from build123d import *

# Parameters (mm, degrees)
ESQUISSE1_W             = 45
ESQUISSE1_H             = 250
BOSS_EXTRU_2_DEPTH      = 3
ESQUISSE2_W             = 3
ESQUISSE2_H             = 250
BOSS_EXTRU_3_DEPTH      = 90
ESQUISSE3_W             = 83
ESQUISSE3_H             = 250
BOSS_EXTRU_4_DEPTH      = 3
ESQUISSE4_R             = 10
ESQUISSE4_R_2           = 2.5
ESQUISSE4_R_3           = 2
ENL_V_MAT_EXTRU_1_DEPTH = 3
ESQUISSE5_R             = 1.5
ENL_V_MAT_EXTRU_2_DEPTH = 3
ENL_V_START             = -3
ESQUISSE6_R             = 10
ESQUISSE6_R_2           = 2
ESQUISSE6_R_3           = 2.5
ENL_V_MAT_EXTRU_3_DEPTH = 3


with BuildPart() as part:
    # Esquisse1 → Boss.-Extru.2 (new body)
    with BuildSketch(Plane.XY):
        with Locations((-2.435511103, -80.979780034)):
            Rectangle(ESQUISSE1_W, ESQUISSE1_H)
    boss_extru_2 = extrude(amount=BOSS_EXTRU_2_DEPTH)

    # Esquisse2 → Boss.-Extru.3 (add)
    with BuildSketch(Plane.XY.offset(3)):
        with Locations((-23.435511103, -80.979780034)):
            Rectangle(ESQUISSE2_W, ESQUISSE2_H)
    boss_extru_3 = extrude(amount=BOSS_EXTRU_3_DEPTH)

    # Esquisse3 → Boss.-Extru.4 (add)
    with BuildSketch(Plane.XY.offset(93)):
        with Locations((-63.435511103, -80.979780034)):
            Rectangle(ESQUISSE3_W, ESQUISSE3_H)
    boss_extru_4 = extrude(amount=BOSS_EXTRU_4_DEPTH)

    # Esquisse4 → Enl_v. mat.-Extru.1 (cut)
    with BuildSketch(Plane.ZY.offset(24.935511103)):
        with Locations(Location((30.5, -80.979780034, 0), (0, 0, 270))):
            Circle(ESQUISSE4_R)
        with Locations(Location((30.5, -59.979780034, 0), (0, 0, 270))):
            Circle(ESQUISSE4_R_2)
        with Locations(Location((48.686533479, -91.479780034, 0), (0, 0, 270))):
            Circle(ESQUISSE4_R_2)
        with Locations(Location((30.5, -0.979780034, 0), (0, 0, 270))):
            Circle(ESQUISSE4_R_3)
        with Locations(Location((30.5, -160.979780034, 0), (0, 0, 270))):
            Circle(ESQUISSE4_R_2)
        with Locations(Location((12.313466521, -91.479780034, 0), (0, 0, 270))):
            Circle(ESQUISSE4_R_2)
    extrude(amount=-ENL_V_MAT_EXTRU_1_DEPTH, mode=Mode.SUBTRACT)

    # Esquisse5 → Enl_v. mat.-Extru.2 (cut)
    with BuildSketch(Plane.XY.offset(96)):
        with BuildLine():
            ThreePointArc((-99.435511103, -80.979780034), (-100.935511103, -79.479780034), (-102.435511103, -80.979780034))
            Line((-102.435511103, -80.979780034), (-99.435511103, -80.979780034))
        make_face()
        with BuildLine():
            Line((-99.435511103, -80.979780034), (-102.435511103, -80.979780034))
            ThreePointArc((-102.435511103, -80.979780034), (-100.935511103, -82.479780034), (-99.435511103, -80.979780034))
        make_face()
        with Locations((-100.935511103, -165.979780034)):
            Circle(ESQUISSE5_R)
        with Locations((-100.935511103, 4.020219966)):
            Circle(ESQUISSE5_R)
    enl_v_mat_extru_2 = extrude(amount=-ENL_V_MAT_EXTRU_2_DEPTH, mode=Mode.SUBTRACT)

    # Sym_trie1: Boss.-Extru.2, Boss.-Extru.3, Boss.-Extru.4, Enl_v. mat.-Extru.2 across plane
    add(boss_extru_2.mirror(Plane(origin=(20.064488897, 44.020219966, 3), x_dir=(0, 0, 1), z_dir=(1, 0, 0))))
    add(boss_extru_3.mirror(Plane(origin=(20.064488897, 44.020219966, 3), x_dir=(0, 0, 1), z_dir=(1, 0, 0))))
    add(boss_extru_4.mirror(Plane(origin=(20.064488897, 44.020219966, 3), x_dir=(0, 0, 1), z_dir=(1, 0, 0))))
    add(enl_v_mat_extru_2.mirror(Plane(origin=(20.064488897, 44.020219966, 3), x_dir=(0, 0, 1), z_dir=(1, 0, 0))), mode=Mode.SUBTRACT)

    # Esquisse6 → Enl_v. mat.-Extru.3 (cut)
    with BuildSketch(Plane(origin=(65.064488897, 0, 0), x_dir=(0, 0, -1), z_dir=(1, 0, 0)).offset(ENL_V_START)):
        with Locations(Location((-30.5, -80.979780034, 0), (0, 0, 270))):
            Circle(ESQUISSE6_R)
        with Locations(Location((-30.5, -0.979780034, 0), (0, 0, 270))):
            Circle(ESQUISSE6_R_2)
        with Locations(Location((-30.5, -160.979780034, 0), (0, 0, 270))):
            Circle(ESQUISSE6_R_3)
        with Locations(Location((-30.5, -101.979780034, 0), (0, 0, 90))):
            Circle(ESQUISSE6_R_3)
        with Locations(Location((-48.686533479, -70.479780034, 0), (0, 0, 90))):
            Circle(ESQUISSE6_R_3)
        with Locations(Location((-12.313466521, -70.479780034, 0), (0, 0, 90))):
            Circle(ESQUISSE6_R_3)
    extrude(amount=ENL_V_MAT_EXTRU_3_DEPTH, mode=Mode.SUBTRACT)


solid = part.part
Can you work these out from the model? Positions are in its coordinate system, mm. A direction names the side the tool comes from. Round coordinates to 2 decimals unless told otherwise and drop trailing zeros. Write each loop counter-clockwise with the first axis right and the second up, starting at its lowest first coordinate (ties: lowest second). Pieces come first, ordered by that corner, then holes. Notation, with made-up numbers: (16, 36.5) -> (43, 36.5) arc R11 ccw to (43, 55.5) -> close; hole circle Ø5 at (71.25, 9). An arc over 180 degrees is marked (long way). Use one line per item in the form item = value. Start each with the question number.
Q1. Imagine slicing it at C-C (x = -81.5). Please give me the cut outline in (y, z), then the cut area to 3 significant figures.
Q2. Imagine slicing it at A-A (z = 84). Please give me the cut outline in (x, y).
Q3. I'm going to push flat-ended pins straight in: P1, Ø6, axis at y = -91.48, z = 12.31, coming from the -X side; P2, Ø10, axis at x = -76, y = -59.5, coming from the -Z side; P3, Ø4.5, axis at y = -59.98, z = 30.5, coming from the -X side; P4, Ø2.5, axis at x = -100.94, y = -165.98, coming from the -Z side. Where does each tip first touch, or does it pass through?
Q4. Imagine slicing it at B-B (y = -150). Please give me the cut outline in (x, z).
Q5. We'd pull the mould along X, two halves only. Please class faces 1 (the face through (65.064, -83, 46)), 2 (the face through (104, -79, 96)), 3 (the face through (21, -79, 3)): +X half, -X half, draft (parallel to the pull), parting line (faces both ways), or undercut.
Q6. If I drill on probe 1 along X at (y, z) = (-32.5, 8.5); probe 2 along Z at (x, y) = (128.5, -188); probe 3 along Z at (x, y) = (-7, -10), over which ranges is the centre line in solid material (lowest first)? Write a range as [from, to].
Q7. Which directions (+Z, -Z, +X, -X, +Y, -Y) give clear straight access to the entire face, cutting with the end or side of a thin tool? Please do faces 4 (the face through (-23.457, -85.594, 21.628)), 5 (the face through (106, -79, 93)), 6 (the face through (-65, -79, 93)), 7 (the face through (62.064, -83, 49)).
Worked out:
q1.outline = (-205.98, 93) -> (44.02, 93) -> (44.02, 96) -> (-205.98, 96) -> close
q1.area = 750 mm^2
q2.outline = (-24.94, -205.98) -> (-21.94, -205.98) -> (-21.94, 44.02) -> (-24.94, 44.02) -> close; (62.06, -205.98) -> (65.06, -205.98) -> (65.06, 44.02) -> (62.06, 44.02) -> close
q3.P1 = -24.94
q3.P2 = 93
q3.P3 = 62.06
q3.P4 = through
q4.outline = (-104.94, 93) -> (-24.94, 93) -> (-24.94, 0) -> (65.06, 0) -> (65.06, 93) -> (145.06, 93) -> (145.06, 96) -> (62.06, 96) -> (62.06, 3) -> (-21.94, 3) -> (-21.94, 96) -> (-104.94, 96) -> close
q5.face_1 = +X half
q5.face_2 = draft
q5.face_3 = undercut
q6.probe_1 = [-24.94, -21.94], [62.06, 65.06]
q6.probe_2 = [93, 96]
q6.probe_3 = [0, 3]
q7.face_4 = +X, -X
q7.face_5 = -Z, +X, +Y, -Y
q7.face_6 = -Z, -X, +Y, -Y
q7.face_7 = +Z, +Y, -Y
